CAD build for the part. Positions are in the model's coordinates, mm. Face numbers are marked on the shaded views. A direction names the side the tool comes from. Round coordinates to 2 decimals unless told otherwise and drop trailing zeros. Order: outer loops, then holes, each group sorted by start corner. A loop starts at its lowest first (then second) coordinate and runs counter-clockwise, first axis right, second up. Notation, with made-up numbers: M -3.5,30 L 17.5,30 A16 ccw 17.5,49 Z; hole C 20.5,58 d11. An arc over 180 degrees is marked long. Answer as a JSON object with one key per item and string values.
```python
from build123d import *

# Parameters (mm, degrees)
F0_R     = 14.2875
F0_W     = 25.4
F0_H     = 50.699268
F1_DEPTH = 2.54
F0_R_2   = 6.35
F2_DEPTH = 3.175


with BuildPart() as f1:
    # F0 (on Front) → F1 (new body)
    with BuildSketch(Plane.XZ):
        Polygon((12.7, 21.997045), (-12.7, 21.997045), (-25.4, 0), (-12.7, -21.997045), (12.7, -21.997045), (25.4, 0), align=None)
        Circle(F0_R, mode=Mode.SUBTRACT)
        with Locations((0, -47.346679)):
            Rectangle(F0_W, F0_H)
    extrude(amount=F1_DEPTH)

    # F0 (on Front) → F2 (join, symmetric)
    with BuildSketch(Plane.XZ):
        Circle(F0_R)
        Circle(F0_R_2, mode=Mode.SUBTRACT)
    extrude(amount=F2_DEPTH, both=True)


solid = f1.part
```
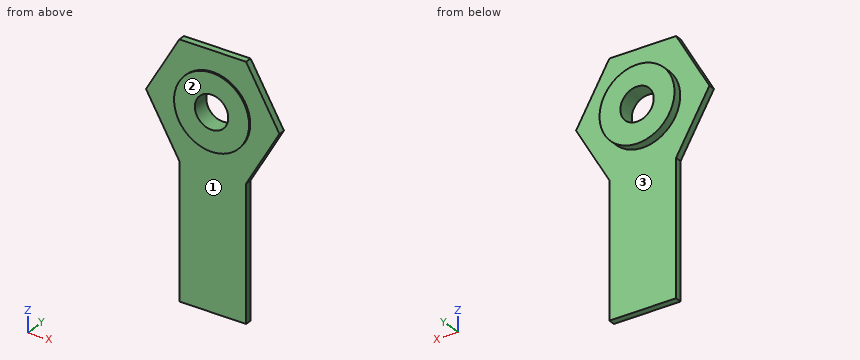
Item 1: Wall check: line 1 along Z through (x, y) = (0, 1.75); line 2 along Z through (x, y) = (0, -0.75); line 3 along Y through (x, z) = (3.5, -42). Give the ranges that are in metal, low to high. Write a range as [from, to].
Worked answers:
{"line 1": "z = [-14.29, -6.35], [6.35, 14.29]", "line 2": "z = [-72.7, -6.35], [6.35, 22]", "line 3": "y = [-2.54, 0]"}
Item 2: Drop flat-ended pins along their axis: pin 1 Ø0.8 at (y, z) = (-1.5, -47.5) entering from -X; pin 2 Ø1.3 at (y, z) = (-1, -42) entering from +X; pin 3 Ø1 at (x, y) = (-2.5, 2.5) entering from +Z. Give the stop position or say it passes through.
Worked answers:
{"pin 1": "stops at x = -12.7", "pin 2": "stops at x = 12.7", "pin 3": "stops at z = 14.15"}
Item 3: 3-axis set-ups, long thin cutter, end or side, ignore diameter. For the marked faces 1, 2 and 3: which of +Z, -Z, +X, -X, +Y, -Y reach the whole face in a straight line?
Worked answers:
{"face 1": "-Y", "face 2": "+Z, -Z, +X, -X, -Y", "face 3": "+Y"}
Item 4: Saw through at D-D on z = -10. List the corners of the cut face in (x, y) (1 decimal), and give its area (3 significant figures).
Worked answers:
{"outline": "M -19.6,-2.5 L -10.2,-2.5 L -10.2,-3.2 L 10.2,-3.2 L 10.2,-2.5 L 19.6,-2.5 L 19.6,0 L 10.2,0 L 10.2,3.2 L -10.2,3.2 L -10.2,0 L -19.6,0 Z", "area": "177 mm2"}
Item 5: Saw through at C-C on z = -33. List the corners of the cut face in (x, y).
Worked answers:
{"outline": "M -12.7,-2.54 L 12.7,-2.54 L 12.7,0 L -12.7,0 Z"}
